Geometry check sheet. Reference: the model listing, model coordinates, mm. A direction names the side the tool comes from. Coordinates: 2 decimals unless noted, no trailing zeros. Order: outer loops, then holes, each group sorted by start corner. A loop starts at its lowest first (then second) coordinate and runs counter-clockwise, first axis right, second up. Notation, with made-up numbers: (37, -13.5) - (87, -13.5) arc R9 ccw to (87, -8.5) - close; hole circle Ø2 at (8, 29.25). An arc over 180 degrees is marked (long way). Use CSV: the item, a comma, the result in double quotes. Start each with the question number.
1) Sectioned sample at A-A, the plane y = 1. Record the cut outline in (x, z) (3 decimals).
2) Sectioned sample at C-C, the plane z = 12. Count the separate pieces of the cut face and the enclosed holes in it, and give its area (3 significant figures).
3) Thickness scan on probe 1 along Y at (x, z) = (-19.5, 1.25); probe 2 along Y at (x, z) = (78.5, 0.75); probe 3 along X at (y, z) = (-11.5, 3). Record the ranges inside material, lowest first. Write a range as [from, to].
4) Depth check by flat-ended pin: P1, Ø11, axis at x = 79.375, y = 34.925, coming from the -Z side (3 decimals). Enter the tip coordinate at first touch or a pass-through.
5) Draft check along Y on faces 1 (the flat face through (34.29, 24, 9)), 2 (the flat face through (88.9, 1, 7)), 3 (the flat face through (1, -44.45, 7)). Enter one of: released by +Y, released by -Y, zero draft, split by the parting line, or undercut.
6) Tool access check on faces 4 (the flat face through (-28, -26.734, 8)), 5 (the flat face through (31.242, 39, 12)), 6 (the flat face through (-88.9, -1, 7)). Record the directions out of +Z, -Z, +X, -X, +Y, -Y that give a thin tool (end or side, any length) a straight path to the whole face; none if there is none.
Autodesk Inventor part; units mm, degrees
ref_plane "Work Plane3" through (51.435, -25.4, 17.145) normal (1, 0, 0) x (0, 0, -1)
ref_plane "Work Plane4" through (33.02, 0, 17.145) normal (0, -1, 0) x (1, 0, 0)
ref_plane "YZ Plane" through (0, 0, 0) normal (1, 0, 0) x (0, 1, 0)
sketch "Sketch1" plane through (0, 0, 0) normal (0, 0, 1) x (1, 0, 0)
  line L0 (88.9, -44.45) -> (-88.9, -44.45)
  line L1 (-88.9, -44.45) -> (-88.9, 44.45)
  line L2 (-88.9, 44.45) -> (88.9, 44.45)
  line L3 (88.9, 44.45) -> (88.9, -44.45)
  line L4 (88.9, -44.45) -> (-88.9, 44.45) construction
  line L5 (-88.9, -44.45) -> (88.9, 44.45) construction
  line L6 (25.4, -26.7335) -> (-82.55, -26.7335)
  line L7 (-82.55, -26.7335) -> (-82.55, 26.7335)
  line L8 (-82.55, 26.7335) -> (25.4, 26.7335)
  line L9 (25.4, 26.7335) -> (25.4, -26.7335)
  line L10 (25.4, -26.7335) -> (-82.55, 26.7335) construction
  line L11 (-82.55, -26.7335) -> (25.4, 26.7335) construction
  line L12 (34.29, 23.1775) -> (20.955, 23.1775)
  line L13 (20.955, 23.1775) -> (20.955, 13.5255)
  line L14 (20.955, 13.5255) -> (34.29, 13.5255)
  line L15 (34.29, 13.5255) -> (34.29, 23.1775)
  line L16 (34.29, 23.1775) -> (20.955, 13.5255) construction
  line L17 (20.955, 23.1775) -> (34.29, 13.5255) construction
  line L18 (23.8125, 33.3375) -> (26.162, 33.3375)
  line L19 (26.162, 33.3375) -> (26.162, 44.45)
  line L20 (31.242, 44.45) -> (31.242, 33.3375)
  line L21 (31.242, 33.3375) -> (34.29, 33.3375)
  line L22 (34.29, 33.3375) -> (34.29, 23.1775)
  line L23 (26.162, 33.3375) -> (31.242, 33.3375) construction
  line L24 (26.162, 44.45) -> (31.242, 44.45)
  line L25 (25.4, 23.1775) -> (34.29, 23.1775)
  line L26 (25.4, 23.1775) -> (25.4, 26.7335)
  line L27 (25.4, 26.7335) -> (25.4, 26.7335)
  line L28 (23.8125, 33.3375) -> (23.8125, 26.7335)
  point P0 (0, 0)
  point P1 (-28.575, 0)
  point P2 (-28.575, 0)
  point P3 (0, 0)
  point P4 (27.6225, 18.3515)
  point P5 (28.702, 33.3375)
  dimension "d0" = 177.8
  dimension "d1" = 88.9
  dimension "d2" = 107.95
  dimension "d3" = 53.467
  dimension "d4" = 6.35
  dimension "d5" = 103.505
  dimension "d7" = 8.382
  dimension "d8" = 9.652
  dimension "d13" = 13.335
  dimension "d15" = 5.08
  dimension "d17" = 10.16
  dimension "d24" = 1.5875
  dimension "d25" = 5.588
extrude "Extrusion1" add sketch "Sketch1" along normal blind 17.145
extrude "Extrusion2" cut sketch "Sketch1" along normal through all contours L20 L21 L22 L12 L9 L8 L28 L18 L19 L2
sketch "Sketch3" plane through (0, 0, 0) normal (0, 0, -1) x (-1, 0, 0)
  line L0 (-31.242, 33.3375) -> (-31.242, 44.45)
  line L1 (-31.242, 44.45) -> (-88.9, 44.45)
  line L2 (-88.9, 44.45) -> (-88.9, -44.45)
  line L3 (-88.9, -44.45) -> (88.9, -44.45)
  line L4 (88.9, -44.45) -> (88.9, 44.45)
  line L5 (88.9, 44.45) -> (-26.162, 44.45)
  line L6 (-26.162, 44.45) -> (-26.162, 33.3375)
  line L7 (-26.162, 33.3375) -> (-23.8125, 33.3375)
  line L8 (-34.29, 23.1775) -> (-34.29, 33.3375)
  line L9 (-34.29, 33.3375) -> (-31.242, 33.3375)
  line L10 (-26.162, 44.45) -> (88.9, 44.45)
  line L11 (-26.162, 44.45) -> (-31.242, 44.45)
  line L12 (-23.8125, 33.3375) -> (-23.8125, 26.7335)
  line L13 (-23.8125, 26.7335) -> (-25.4, 26.7335)
  line L14 (-25.4, 26.7335) -> (-25.4, 23.1775)
  line L15 (-25.4, 23.1775) -> (-34.29, 23.1775)
  point P0 (0, 0)
extrude "Extrusion4" add sketch "Sketch3" along normal blind 3.175
ref_plane "Work Plane1" through (-28.575, -26.7335, 12.7) normal (1, 0, 0) x (0, 0, -1)
ref_plane "Work Plane2" through (-82.55, 0, 12.7) normal (0, -1, 0) x (1, 0, 0)
sketch "Sketch5" plane through (0, 0, 17.145) normal (0, 0, 1) x (1, 0, 0)
  line L0 (69.85, -25.4) -> (33.02, -25.4)
  line L1 (33.02, -25.4) -> (33.02, 25.4)
  line L2 (33.02, 25.4) -> (69.85, 25.4)
  line L3 (69.85, 25.4) -> (69.85, -25.4)
  line L4 (69.85, -25.4) -> (33.02, 25.4) construction
  line L5 (33.02, -25.4) -> (69.85, 25.4) construction
  line L6 (124.46, 0) -> (-124.46, 0)
  line L7 (88.9, -44.45) -> (88.9, 44.45)
  line L8 (69.85, 25.4) -> (63.5, 25.4)
  line L9 (63.5, 25.4) -> (63.5, 44.45)
  line L10 (63.5, 44.45) -> (69.85, 44.45)
  line L11 (69.85, 44.45) -> (69.85, 25.4)
  line L12 (88.9, 44.45) -> (-88.9, 44.45)
  point P0 (0, 0)
  point P1 (51.435, 0)
  point P2 (51.435, 0)
  point P3 (31.242, 44.45)
  dimension "d26" = 36.83
  dimension "d27" = 50.8
  dimension "d28" = 19.05
  dimension "d29" = 6.35
extrude "Extrusion5" cut sketch "Sketch5" against normal up to surface (17.145 mm away) contours L0 L1 L6 L3 | L6 L1 L2 L3 | L2 L9 L10 L11
ref_plane "Work Plane3" through (51.435, -25.4, 17.145) normal (1, 0, 0) x (0, 0, -1)
ref_plane "Work Plane4" through (33.02, 0, 17.145) normal (0, -1, 0) x (1, 0, 0)
sketch "Sketch6" plane through (0, 0, 17.145) normal (0, 0, 1) x (1, 0, 0)
  line L0 (69.85, 44.45) -> (69.85, -25.4)
  line L1 (69.85, -25.4) -> (33.02, -25.4)
  line L2 (33.02, -25.4) -> (33.02, 23.1775)
  line L3 (34.29, 25.4) -> (63.5, 25.4)
  line L4 (63.5, 25.4) -> (63.5, 44.45)
  line L5 (26.162, 44.45) -> (-88.9, 44.45)
  line L6 (-88.9, 44.45) -> (-88.9, -44.45)
  line L7 (-88.9, -44.45) -> (88.9, -44.45)
  line L8 (88.9, -44.45) -> (88.9, 44.45)
  line L9 (88.9, 44.45) -> (69.85, 44.45)
  line L10 (33.02, -25.4) -> (33.02, 25.4)
  line L11 (39.37, 25.4) -> (63.5, 25.4)
  line L12 (63.5, 25.4) -> (63.5, 38.1)
  line L13 (63.5, 38.1) -> (39.37, 38.1)
  line L14 (39.37, 38.1) -> (39.37, 25.4)
  line L15 (39.37, 38.1) -> (33.02, 38.1)
  line L16 (33.02, 38.1) -> (33.02, 25.4)
  line L17 (33.02, 25.4) -> (39.37, 25.4)
  line L18 (36.195, 25.4) -> (36.195, -22.225)
  line L19 (33.02, 25.4) -> (33.02, -19.05)
  line L20 (33.02, -19.05) -> (25.4, -19.05)
  line L21 (25.4, -26.7335) -> (25.4, 13.5255)
  line L22 (36.195, -22.225) -> (25.4, -22.225)
  line L23 (25.4, -19.05) -> (25.4, -22.225)
  line L24 (63.5, 44.45) -> (31.242, 44.45)
  line L25 (31.242, 44.45) -> (31.242, 33.3375)
  line L26 (31.242, 33.3375) -> (34.29, 33.3375)
  line L27 (34.29, 33.3375) -> (34.29, 25.4)
  line L28 (33.02, 23.1775) -> (25.4, 23.1775)
  line L29 (25.4, 23.1775) -> (25.4, 26.7335)
  line L30 (25.4, 26.7335) -> (23.8125, 26.7335)
  line L31 (23.8125, 26.7335) -> (23.8125, 33.3375)
  line L32 (23.8125, 33.3375) -> (26.162, 33.3375)
  line L33 (26.162, 33.3375) -> (26.162, 44.45)
  point P0 (0, 0)
  dimension "d32" = 12.7
  dimension "d33" = 3.175
  dimension "d34" = 3.175
  dimension "d35" = 22.225
extrude "Extrusion6" cut sketch "Sketch6" against normal blind 9.525 contours L14 L13 L4 L3
extrude "Extrusion7" cut sketch "Sketch6" against normal blind 9.525 contours L22 L21 L20 L2 | L2 L10 L17 L3 L18 L22 | L3 L27 L26 L16 L15 L14 | L16 L26 L27 L17
sketch "Sketch7" plane through (0, 0, 0) normal (0, 0, 1) x (1, 0, 0)
  line L0 (26.162, 44.45) -> (26.162, 33.3375)
  line L1 (26.162, 33.3375) -> (23.8125, 33.3375)
  line L2 (23.8125, 33.3375) -> (23.8125, 26.7335)
  line L3 (34.29, 25.4) -> (34.29, 33.3375)
  line L4 (34.29, 33.3375) -> (31.242, 33.3375)
  line L5 (31.242, 33.3375) -> (31.242, 44.45)
  line L6 (26.162, 44.45) -> (31.242, 44.45)
  line L7 (26.162, 33.3375) -> (26.162, 44.45)
  line L8 (26.162, 33.3375) -> (31.242, 33.3375)
  line L9 (23.8125, 26.7335) -> (25.4, 26.7335)
  line L10 (25.4, 26.7335) -> (25.4, 23.1775)
  line L11 (25.4, 23.1775) -> (33.02, 23.1775)
  line L12 (33.02, -25.4) -> (33.02, 23.1775)
  line L13 (69.85, -25.4) -> (33.02, -25.4)
  line L14 (69.85, 44.45) -> (69.85, -25.4)
  line L15 (63.5, 44.45) -> (69.85, 44.45)
  line L16 (63.5, 25.4) -> (63.5, 44.45)
  line L17 (34.29, 25.4) -> (63.5, 25.4)
  point P0 (0, 0)
extrude "Extrusion8" add sketch "Sketch7" along normal blind 6.35 contours L6 L5 L8 L0
extrude "Extrusion9" cut sketch "Sketch1" along normal through all contours L8 L9 L12 L13 L14 L6 L7 | L9 L14 L13 L12
sketch "Sketch8" plane through (0, 0, 17.145) normal (0, 0, 1) x (1, 0, 0)
  line L0 (20.955, 13.5255) -> (34.29, 13.5255)
  line L1 (20.955, 23.1775) -> (20.955, 13.5255)
  line L2 (34.29, 23.1775) -> (20.955, 23.1775)
  line L3 (34.29, 13.5255) -> (34.29, 23.1775)
  point P0 (0, 0)
extrude "Extrusion10" cut sketch "Sketch8" against normal up to surface (17.145 mm away)
sketch "Sketch10" plane through (0, 0, -3.175) normal (0, 0, -1) x (-1, 0, 0)
  circle A0 centre (-79.375, 34.925) radius 3.3782
  circle A1 centre (79.375, -34.925) radius 3.3782
  circle A2 centre (79.375, 34.925) radius 3.3782
  circle A3 centre (-79.375, -34.925) radius 3.3782
  line L0 (88.9, 44.45) -> (-88.9, 44.45)
  line L1 (-88.9, 44.45) -> (-88.9, -44.45)
  line L2 (-88.9, -44.45) -> (88.9, -44.45)
  line L3 (88.9, -44.45) -> (88.9, 44.45)
  point P0 (0, 0)
extrude "Extrusion11" cut sketch "Sketch10" against normal through all contours A0 | A1 | A2 | A3
sketch "Sketch12" plane through (0, 0, 17.145) normal (0, 0, 1) x (1, 0, 0)
  circle A0 centre (-79.375, 34.925) radius 3.3782
  circle A1 centre (79.375, 34.925) radius 3.3782
  circle A2 centre (-79.375, -34.925) radius 3.3782
  circle A3 centre (79.375, -34.925) radius 3.3782
  line L0 (-82.55, 26.7335) -> (23.8125, 26.7335)
  line L1 (23.8125, 26.7335) -> (23.8125, 33.3375)
  line L2 (23.8125, 33.3375) -> (26.162, 33.3375)
  line L3 (26.162, 33.3375) -> (26.162, 44.45)
  line L4 (26.162, 44.45) -> (-88.9, 44.45)
  line L5 (-88.9, 44.45) -> (-88.9, -44.45)
  line L6 (-88.9, -44.45) -> (88.9, -44.45)
  line L7 (88.9, -44.45) -> (88.9, 44.45)
  line L8 (88.9, 44.45) -> (69.85, 44.45)
  line L9 (69.85, 44.45) -> (69.85, -25.4)
  line L10 (69.85, -25.4) -> (33.02, -25.4)
  line L11 (33.02, -25.4) -> (33.02, -22.225)
  line L12 (33.02, -22.225) -> (25.4, -22.225)
  line L13 (25.4, -22.225) -> (25.4, -26.7335)
  line L14 (25.4, -26.7335) -> (-82.55, -26.7335)
  line L15 (-82.55, -26.7335) -> (-82.55, 26.7335)
  line L16 (33.02, 13.5255) -> (25.4, 13.5255)
  line L17 (69.85, 44.45) -> (69.85, -25.4)
  line L18 (25.4, 13.5255) -> (69.85, 13.5255)
  line L19 (69.85, 13.5255) -> (69.85, -25.4)
  line L20 (69.85, -25.4) -> (25.4, -25.4)
  line L21 (25.4, -25.4) -> (25.4, 13.5255)
  line L22 (33.02, 33.3375) -> (33.02, 38.1)
  line L23 (33.02, 38.1) -> (33.02, 33.3375)
  line L24 (33.02, 33.3375) -> (69.85, 33.3375)
  line L25 (69.85, 33.3375) -> (69.85, 38.1)
  line L26 (69.85, 38.1) -> (33.02, 38.1)
  line L27 (69.85, 33.3375) -> (34.29, 33.3375)
  line L28 (34.29, 33.3375) -> (34.29, 13.5255)
  line L29 (34.29, 13.5255) -> (69.85, 13.5255)
  line L30 (69.85, 13.5255) -> (69.85, 33.3375)
  line L31 (63.5, 44.45) -> (69.85, 44.45)
  line L32 (69.85, 44.45) -> (69.85, 38.1)
  line L33 (69.85, 38.1) -> (63.5, 38.1)
  line L34 (63.5, 38.1) -> (63.5, 44.45)
  point P0 (0, 0)
extrude "Extrusion12" add sketch "Sketch12" against normal up to surface (17.145 mm away) contours L13 L12 L11 L20 | L21 L16 L18 L9 L10 L11 L12 | L18 L28 L24 L9 | L24 L22 L26 L9 | L26 L34 L31 L9
sketch "Sketch9" plane through (0, 0, -3.175) normal (0, 0, -1) x (-1, 0, 0)
  point P0 (79.375, -34.925)
  point P1 (79.375, 34.925)
  point P2 (-79.375, 34.925)
  point P3 (-79.375, -34.925)
equation "\"d34\" = d33"
properties part number "ArduinPanel2"
Evaluation:
1,outline,"(-88.9, -3.175) - (88.9, -3.175) - (88.9, 17.145) - (25.4, 17.145) - (25.4, 0) - (-82.55, 0) - (-82.55, 17.145) - (-88.9, 17.145) - close"
2,separate pieces,"1"
2,enclosed holes,"4"
2,area,"9,650 mm²"
3,probe 1,"[-44.45, -26.73], [26.73, 44.45]"
3,probe 2,"[-44.45, -38.19], [-31.66, 31.66], [38.19, 44.45]"
3,probe 3,"[-88.9, -82.55], [25.4, 88.9]"
4,P1,"z = -3.175"
5,face 1,"undercut"
5,face 2,"zero draft"
5,face 3,"released by -Y"
6,face 4,"+Z"
6,face 5,"+Z, +Y"
6,face 6,"+Z, -Z, -X, +Y, -Y"
